Input: part model. Units: mm. Frame: model coordinates. Coordinates: 2 decimals unless noted, no trailing zeros. Order: outer loops, then holes, each group sorted by start corner. A loop starts at its lowest first (then second) coordinate and runs counter-clockwise, first axis right, second up. Notation, with made-up numbers: M 7.5,43.25 L 36.5,43.25 A27 cw 36.5,62.25 Z; hole C -5,85.5 d5. An arc over 180 degrees is marked long. One line per item, written item: value.
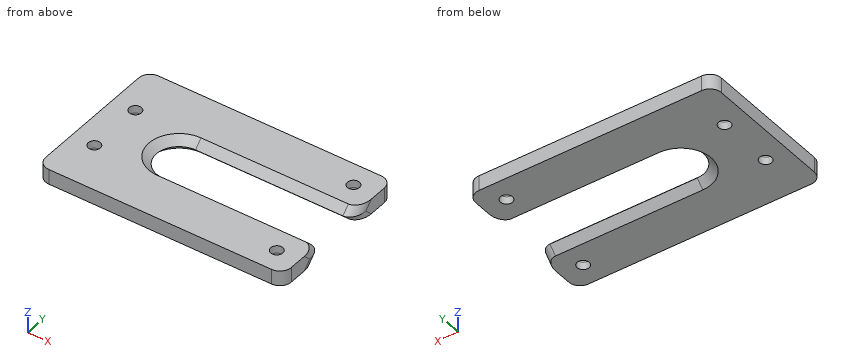
```python
from build123d import *

# Parameters (mm, degrees)
PAD_DEPTH         = 65
SKETCH009_R       = 1.6
POCKET_DEPTH      = 2.001
POCKET_DEPTH_BACK = 2.001
SKETCH004_R       = 8
SKETCH003_R       = 6
SKETCH005_R       = 8
FILLET_R          = 3
FILLET001_R       = 3


with BuildPart() as part:
    # Sketch → Pad (new body)
    with BuildSketch(Plane.YZ):
        Polygon((0, 2), (-20, 2), (-20, 0), (-20, -2), (0, -2), (20, -2), (20, 0), (20, 2), align=None)
    extrude(amount=PAD_DEPTH)

    # Sketch009 → Pocket (cut, two sides)
    with BuildSketch(Plane.XY) as pocket_sk:
        with Locations((6, 7.5)):
            Circle(SKETCH009_R)
        with Locations((6, -7.5)):
            Circle(SKETCH009_R)
        with Locations((59, -14)):
            Circle(SKETCH009_R)
        with Locations((59, 14)):
            Circle(SKETCH009_R)
    extrude(amount=-POCKET_DEPTH, mode=Mode.SUBTRACT)
    extrude(pocket_sk.sketch, amount=POCKET_DEPTH_BACK, mode=Mode.SUBTRACT)

    # Sketch004 (on DatumPlane) → SubtractiveLoft section 0
    with BuildSketch(Plane.XY.offset(2)):
        with Locations((23, 0)):
            Circle(SKETCH004_R)
    # Sketch003 → SubtractiveLoft section 1
    with BuildSketch(Plane.XY):
        with Locations((23, 0)):
            Circle(SKETCH003_R)
    # Sketch005 (on DatumPlane) → SubtractiveLoft section 2
    with BuildSketch(Plane.XY.offset(-2)):
        with Locations((23, 0)):
            Circle(SKETCH005_R)
    loft(ruled=True, mode=Mode.SUBTRACT)

    # Sketch007 (on DatumPlane) → SubtractiveLoft001 section 0
    with BuildSketch(Plane.XY.offset(2)):
        Polygon((23, 0), (23, 8), (123, 8), (123, -8), (23, -8), align=None)
    # Sketch006 → SubtractiveLoft001 section 1
    with BuildSketch(Plane.XY):
        Polygon((23, 0), (23, 6), (123, 6), (123, -6), (23, -6), align=None)
    # Sketch008 (on DatumPlane) → SubtractiveLoft001 section 2
    with BuildSketch(Plane.XY.offset(-2)):
        Polygon((23, 8), (23, 0), (23, -8), (123, -8), (123, 8), align=None)
    loft(ruled=True, mode=Mode.SUBTRACT)

    # Fillet
    fillet_edges = [part.edges().sort_by_distance(p)[0] for p in [
        (65, -20, 1),
        (0, -20, 1),
        (0, 20, 1),
        (65, 20, 1),
    ]]
    fillet(fillet_edges, radius=FILLET_R)

    # Fillet001
    fillet001_edges = [part.edges().sort_by_distance(p)[0] for p in [
        (65, -7, 1),
        (65, -7, -1),
        (65, 7, -1),
        (65, 7, 1),
    ]]
    fillet(fillet001_edges, radius=FILLET001_R)


solid = part.part
```
(1) Cut plane A-A on x = 59. Output: boundary loops of the cut face in (y, z), plus the area to 3 significant figures.
Data:
outline: M -20,-2 L -15.6,-2 L -15.6,2 L -20,2 Z; M -12.4,-2 L -8,-2 L -6,0 L -8,2 L -12.4,2 Z; M 6,0 L 8,-2 L 12.4,-2 L 12.4,2 L 8,2 Z; M 15.6,-2 L 20,-2 L 20,2 L 15.6,2 Z
area: 78.4 mm2
(2) Ray query, line 1 (Y direction, x = 6, z = 1.3); line 2 (Y direction, x = 59.5, z = 1.3); line 3 (Y direction, x = 59, z = 0.75). Return the intervals inside material, ascending. Write a range as from..to.
Data:
line 1: y = -20..-9.1, -5.9..5.9, 9.1..20
line 2: y = -20..-15.52, -12.48..-7.3, 7.3..12.48, 15.52..20
line 3: y = -20..-15.6, -12.4..-6.75, 6.75..12.4, 15.6..20
(3) Cut plane C-C on x = 6. Output: boundary loops of the cut face in (y, z).
Data:
outline: M -20,-2 L -9.1,-2 L -9.1,2 L -20,2 Z; M -5.9,-2 L 5.9,-2 L 5.9,2 L -5.9,2 Z; M 9.1,-2 L 20,-2 L 20,2 L 9.1,2 Z
(4) First-contact query: pin 1 (3 mm diameter, centred on x = 59, y = 14, fed in from +Z); pin 2 (3.5 mm diameter, centred on x = 6, y = 7.5, fed in from -Z). Flat tips, straight axial feed; report the tip coordinate or a pass-through.
Data:
pin 1: passes through
pin 2: stops at z = -2
(5) Cut plane B-B on y = -14. Output: boundary loops of the cut face in (x, z), plus the area to 3 significant figures.
Data:
outline: M 0,-2 L 57.4,-2 L 57.4,2 L 0,2 Z; M 60.6,-2 L 65,-2 L 65,2 L 60.6,2 Z
area: 247 mm2
(6) Cut plane D-D on x = 34.5. Output: boundary loops of the cut face in (y, z), plus the area to 3 significant figures.
Data:
outline: M -20,-2 L -8,-2 L -6,0 L -8,2 L -20,2 Z; M 6,0 L 8,-2 L 20,-2 L 20,2 L 8,2 Z
area: 104 mm2
